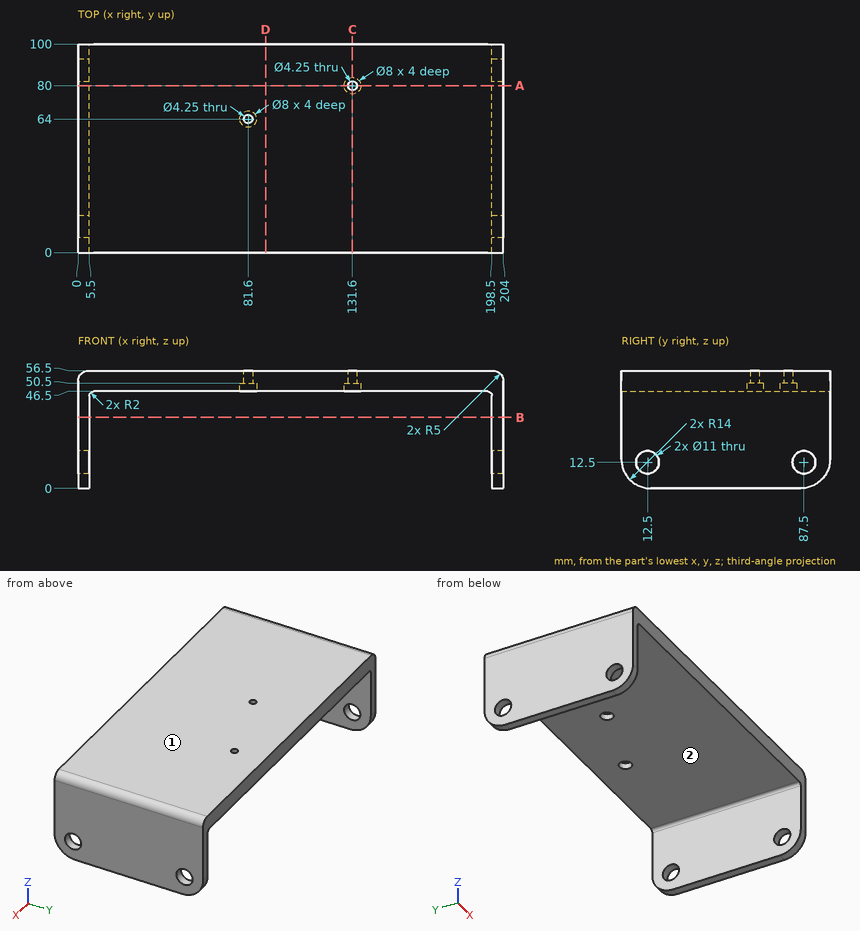
Drawing for the job (mm, zero at the part's lowest x, y, z). A direction names the side the tool comes from. Round coordinates to 2 decimals unless told otherwise and drop trailing zeros. Write each loop counter-clockwise with the first axis right and the second up, starting at its lowest first coordinate (ties: lowest second). Pieces come first, ordered by that corner, then holes. Notation, with made-up numbers: (82, 80.25) - (93, 80.25) arc R28 cw to (93, 109.25) - close; hole circle Ø1 at (42, 7). An arc over 180 degrees is marked (long way). Write item = value, one per line. Start each with the question number.
Q1. Which spindle directions (+Z, -Z, +X, -X, +Y, -Y) get a long thin tool onto all of the face, cutting with end or side? Do the marked faces 1 and 2. Say none if no direction does.
Q2. Band-saw the part on A-A (y = 80). Give the cut face in (x, z) (3 decimals), then the cut area to 3 significant figures.
Q3. Band-saw the part on C-C (x = 131.6). Give the cut face in (y, z) (3 decimals), then the cut area to 4 significant figures.
Q4. Band-saw the part on D-D (x = 90). Give the cut face in (y, z), then the cut area to 3 significant figures.
Q5. Drop flat-ended pins along their axis: pin 1 (1 mm diameter, centred on x = 163, y = 63, fed in from -Z); pin 2 (7 mm diameter, centred on x = 131.6, y = 80, fed in from -Z); pin 3 (12.5 mm diameter, centred on y = 12.5, z = 12.5, fed in from -X). Give the stop position or say it passes through.
Q6. Probe L1, parallel to X at y = 51, z = 13; L2, parallel to Z at x = 155.5, y = 21; L3, parallel to Y at x = 131.6, z = 47.75. List the from-to ranges inside material, lowest first. Write a range as from..to.
Q7. Band-saw the part on B-B (z = 34). Give the cut face in (x, y).
Answers below:
q1.face_1 = +Z, +X, -X, +Y, -Y
q1.face_2 = -Z, +Y, -Y
q2.outline = (0, 0) - (5.5, 0) - (5.5, 44.5) arc R2 cw to (7.5, 46.5) - (127.6, 46.5) - (127.6, 50.5) - (129.475, 50.5) - (129.475, 56.5) - (5, 56.5) arc R5 ccw to (0, 51.5) - close; (133.725, 50.5) - (135.6, 50.5) - (135.6, 46.5) - (196.5, 46.5) arc R2 cw to (198.5, 44.5) - (198.5, 0) - (204, 0) - (204, 51.5) arc R5 ccw to (199, 56.5) - (133.725, 56.5) - close
q2.area = 2,480 mm2
q3.outline = (0, 46.5) - (76, 46.5) - (76, 50.5) - (77.875, 50.5) - (77.875, 56.5) - (0, 56.5) - close; (82.125, 50.5) - (84, 50.5) - (84, 46.5) - (100, 46.5) - (100, 56.5) - (82.125, 56.5) - close
q3.area = 942.5 mm2
q4.outline = (0, 46.5) - (100, 46.5) - (100, 56.5) - (0, 56.5) - close
q4.area = 1,000 mm2
q5.pin_1 = 46.5
q5.pin_2 = 50.5
q5.pin_3 = 0
q6.L1 = 0..5.5, 198.5..204
q6.L2 = 46.5..56.5
q6.L3 = 0..76, 84..100
q7.outline = (0, 0) - (5.5, 0) - (5.5, 100) - (0, 100) - close; (198.5, 0) - (204, 0) - (204, 100) - (198.5, 100) - close
